CAD build for the part. Positions are in the model's coordinates, mm. Face numbers are marked on the shaded views. Give positions to 0.01 mm unless a question says otherwise; leave off trailing zeros. Loops run counter-clockwise (first coordinate to the right, second up) from the corner with the lowest first, then second, coordinate; pieces in that order, holes last. Notation, with made-up numbers: M 4.25,-9 L 60.25,-9 A27 cw 60.25,11 Z; hole C 72,-8 d8. An arc over 180 degrees is marked long. Answer as CSV lines item,"result".
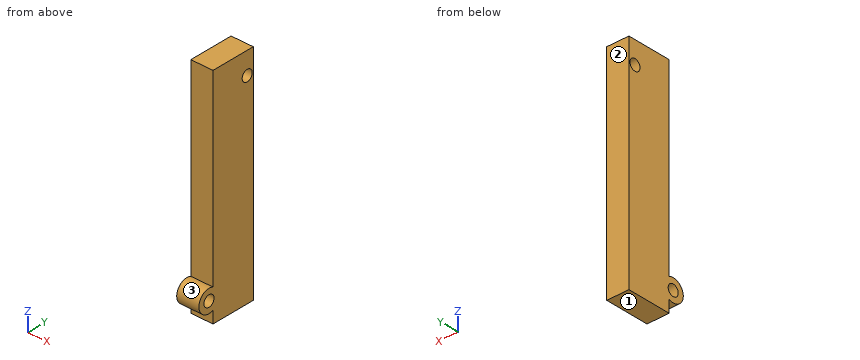
Autodesk Inventor part; units mm, degrees
ref_plane "YZ Plane" through (0, 0, 0) normal (1, 0, 0) x (0, 1, 0)
ref_plane "XZ Plane" through (0, 0, 0) normal (0, 1, 0) x (-1, 0, 0)
ref_plane "XY Plane" through (0, 0, 0) normal (0, 0, 1) x (1, 0, 0)
sketch "Sketch1" plane through (0, 0, 0) normal (1, 0, 0) x (0, 1, 0)
  line L0 (-10, 50) -> (10, 50)
  line L1 (10, 50) -> (10, -50)
  line L2 (10, -50) -> (-10, -50)
  line L3 (-10, -50) -> (-10, 50)
  line L4 (-10, 50) -> (10, -50) construction
  line L5 (10, 50) -> (-10, -50) construction
  circle A0 centre (7, 40) radius 2.5
  circle A1 centre (7, 40) radius 5
  circle A2 centre (-12, -40) radius 2.5
  circle A3 centre (-12, -40) radius 5
  point P0 (0, 0)
  point P1 (0, 0)
  point P2 (-10, 35.4174)
  point P3 (-10, -35.4174)
  point P4 (-10, -44.5826)
  point P5 (-10, 44.5826)
  point P6 (10, 36)
  point P7 (10, 44)
  point P8 (-10, -38.5)
  point P9 (-10, -41.5)
  dimension "d0" = 100
  dimension "d1" = 5
  dimension "d2" = 10
  dimension "d3" = 10
  dimension "d5" = 20
  dimension "d6" = 5
  dimension "d7" = 10
  dimension "d8" = 2
  dimension "d9" = 10
  dimension "d12" = 3
extrude "Extrusion1" add sketch "Sketch1" along normal blind 10 contours L0 L1 A1 L2 L3 A3 | A3 L3 A2 | L3 A2 A3 | L1 A1 picked at (9.8333, 40)
properties part number "temp-bed"
Q1. Pin check, flat tips, straight feed: P1, Ø3, axis at x = 7.5, z = 4.5, coming from the -Y side; P2, Ø3, axis at y = -12, z = -40, coming from the +X side. Stop position of each tip, or through.
Solution:
P1,"stops at y = -10"
P2,"passes through"
Q2. Cut at A-A (z = -40). Write the cut outline in (x, y).
Solution:
outline,"M 0,-17 L 10,-17 L 10,-14.5 L 0,-14.5 Z; M 0,-9.5 L 10,-9.5 L 10,10 L 0,10 Z"
Q3. Cut at C-C (y = -12). Write the cut outline in (x, z), and give its area (3 significant figures).
Solution:
outline,"M 0,-45 L 10,-45 L 10,-42.5 L 0,-42.5 Z; M 0,-37.5 L 10,-37.5 L 10,-35 L 0,-35 Z"
area,"50.0 mm²"
Q4. Mould opens along Y. For the marked faces 1, 2 and 3 say: released by +Y, released by -Y, zero draft, split by the parting line, or undercut.
Solution:
face 1,"zero draft"
face 2,"released by +Y"
face 3,"undercut"
Q5. Cut at B-B (x = 9). Write the cut outline in (y, z), and give its area (3 significant figures).
Solution:
outline,"M -10,-50 L 10,-50 L 10,50 L -10,50 L -10,-35.42 A5 ccw long -10,-44.58 Z; hole C -12,-40 d5; hole C 7,40 d5"
area,"2,020 mm²"
Q6. Cut at D-D (z = 7.5). Write the cut outline in (x, y).
Solution:
outline,"M 0,-10 L 10,-10 L 10,10 L 0,10 Z"
Q7. Wall check: line 1 (Y direction, x = 4.25, z = -40); line 2 (Z direction, x = 4.75, y = 7); line 3 (Z direction, x = 4.5, y = -12). Give the ranges that are in metal, low to high. Write a range as [from, to].
Solution:
line 1,"y = [-17, -14.5], [-9.5, 10]"
line 2,"z = [-50, 37.5], [42.5, 50]"
line 3,"z = [-45, -42.5], [-37.5, -35]"
